from build123d import *

# Parameters (mm, degrees)
BOSS_EXTRUDE1_DEPTH = 3.6
BOSS_EXTRUDE2_DEPTH = 1.5
CUT_EXTRUDE1_DEPTH  = 3.6
BOSS_EXTRUDE5_DEPTH = 3.6
CHAMFER1_SIZE       = 3.6
CHAMFER1_SIZE_2     = 0.062838234
FILLET3_R           = 1
CHAMFER2_SIZE       = 0.6
FILLET4_R           = 0.8


with BuildPart() as part:
    # Sketch1 → Boss-Extrude1 (new body)
    with BuildSketch(Plane(origin=(0, 0, 0), x_dir=(1, 0, 0), z_dir=(0, 1, 0))):
        with BuildLine():
            Line((6, 0), (26.9, 0))
            ThreePointArc((26.9, 0), (31.142640687, 1.757359313), (32.9, 6))
            Line((32.9, 6), (32.9, 17.9))
            ThreePointArc((32.9, 17.9), (31.142640687, 22.142640687), (26.9, 23.9))
            Line((26.9, 23.9), (6, 23.9))
            ThreePointArc((6, 23.9), (1.757359313, 22.142640687), (0, 17.9))
            Line((0, 17.9), (0, 6))
            ThreePointArc((0, 6), (1.757359313, 1.757359313), (6, 0))
        make_face()
    extrude(amount=BOSS_EXTRUDE1_DEPTH)

    # Sketch2 → Boss-Extrude2 (add)
    with BuildSketch(Plane(origin=(0, 3.6, 0), x_dir=(1, 0, 0), z_dir=(0, 1, 0))):
        with BuildLine():
            Line((4.75, 25.15), (28.15, 25.15))
            ThreePointArc((28.15, 25.15), (32.392640687, 23.392640687), (34.15, 19.15))
            Line((34.15, 19.15), (34.15, 4.75))
            ThreePointArc((34.15, 4.75), (32.392640687, 0.507359313), (28.15, -1.25))
            Line((28.15, -1.25), (4.75, -1.25))
            ThreePointArc((4.75, -1.25), (0.507359313, 0.507359313), (-1.25, 4.75))
            Line((-1.25, 4.75), (-1.25, 19.15))
            ThreePointArc((-1.25, 19.15), (0.507359313, 23.392640687), (4.75, 25.15))
        make_face()
    extrude(amount=BOSS_EXTRUDE2_DEPTH)

    # Sketch3 → Cut-Extrude1 (cut)
    with BuildSketch(Plane.XZ):
        with BuildLine():
            Line((25.7, -22.7), (7.2, -22.7))
            ThreePointArc((7.2, -22.7), (2.957359313, -20.942640687), (1.2, -16.7))
            Line((1.2, -16.7), (1.2, -7.2))
            ThreePointArc((1.2, -7.2), (2.957359313, -2.957359313), (7.2, -1.2))
            Line((7.2, -1.2), (25.7, -1.2))
            ThreePointArc((25.7, -1.2), (29.942640687, -2.957359313), (31.7, -7.2))
            Line((31.7, -7.2), (31.7, -16.7))
            ThreePointArc((31.7, -16.7), (29.942640687, -20.942640687), (25.7, -22.7))
        make_face()
    extrude(amount=-CUT_EXTRUDE1_DEPTH, mode=Mode.SUBTRACT)

    # Sketch5 → Boss-Extrude5 (add)
    with BuildSketch(Plane.XZ.offset(-3.6)):
        with BuildLine():
            Line((7.2, -1.2), (8.4, -1.2))
            Line((8.4, -1.2), (8.4, -6.2))
            ThreePointArc((8.4, -6.2), (8.692893219, -6.907106781), (9.4, -7.2))
            Line((9.4, -7.2), (23.5, -7.2))
            ThreePointArc((23.5, -7.2), (24.207106781, -6.907106781), (24.5, -6.2))
            Line((24.5, -6.2), (24.5, -1.2))
            Line((24.5, -1.2), (25.7, -1.2))
            Line((25.7, -1.2), (25.7, -6.2))
            ThreePointArc((25.7, -6.2), (25.992893219, -6.907106781), (26.7, -7.2))
            Line((26.7, -7.2), (31.7, -7.2))
            Line((31.7, -7.2), (31.7, -8.4))
            Line((31.7, -8.4), (26.7, -8.4))
            ThreePointArc((26.7, -8.4), (25.992893219, -8.692893219), (25.7, -9.4))
            Line((25.7, -9.4), (25.7, -14.5))
            ThreePointArc((25.7, -14.5), (25.992893219, -15.207106781), (26.7, -15.5))
            Line((26.7, -15.5), (31.7, -15.5))
            Line((31.7, -15.5), (31.7, -16.7))
            Line((31.7, -16.7), (26.7, -16.7))
            ThreePointArc((26.7, -16.7), (25.992893219, -16.992893219), (25.7, -17.7))
            Line((25.7, -17.7), (25.7, -22.7))
            Line((25.7, -22.7), (24.5, -22.7))
            Line((24.5, -22.7), (24.5, -17.7))
            ThreePointArc((24.5, -17.7), (24.207106781, -16.992893219), (23.5, -16.7))
            Line((23.5, -16.7), (9.4, -16.7))
            ThreePointArc((9.4, -16.7), (8.692893219, -16.992893219), (8.4, -17.7))
            Line((8.4, -17.7), (8.4, -22.7))
            Line((8.4, -22.7), (7.2, -22.7))
            Line((7.2, -22.7), (7.2, -17.7))
            ThreePointArc((7.2, -17.7), (6.907106781, -16.992893219), (6.2, -16.7))
            Line((6.2, -16.7), (1.2, -16.7))
            Line((1.2, -16.7), (1.2, -15.5))
            Line((1.2, -15.5), (6.2, -15.5))
            ThreePointArc((6.2, -15.5), (6.907106781, -15.207106781), (7.2, -14.5))
            Line((7.2, -14.5), (7.2, -9.4))
            ThreePointArc((7.2, -9.4), (6.907106781, -8.692893219), (6.2, -8.4))
            Line((6.2, -8.4), (1.2, -8.4))
            Line((1.2, -8.4), (1.2, -7.2))
            Line((1.2, -7.2), (6.2, -7.2))
            ThreePointArc((6.2, -7.2), (6.907106781, -6.907106781), (7.2, -6.2))
            Line((7.2, -6.2), (7.2, -1.2))
        make_face()
        with BuildLine():
            Line((9.4, -8.4), (23.5, -8.4))
            ThreePointArc((23.5, -8.4), (24.207106781, -8.692893219), (24.5, -9.4))
            Line((24.5, -9.4), (24.5, -14.5))
            ThreePointArc((24.5, -14.5), (24.207106781, -15.207106781), (23.5, -15.5))
            Line((23.5, -15.5), (9.4, -15.5))
            ThreePointArc((9.4, -15.5), (8.692893219, -15.207106781), (8.4, -14.5))
            Line((8.4, -14.5), (8.4, -9.4))
            ThreePointArc((8.4, -9.4), (8.692893219, -8.692893219), (9.4, -8.4))
        make_face(mode=Mode.SUBTRACT)
    extrude(amount=BOSS_EXTRUDE5_DEPTH)

    # Chamfer1
    # the kernel refuses this chamfer: 3.6, 0.062838234 mm, written as the material it takes off along each edge
    with BuildSketch(Plane(origin=(0, 0, -17.9), x_dir=(-0.0006712501823120534, 0.9999997747115711, 0), z_dir=(0, 0, 1))) as chamfer1_piece_1_section:
        Polygon((CHAMFER1_SIZE * 0.999999774712, -CHAMFER1_SIZE * 0.000671250182312), (-CHAMFER1_SIZE_2 * 0.000671250179552, -CHAMFER1_SIZE_2 * 0.999999770599), (0, 0), align=None)
    chamfer1_piece_1 = extrude(amount=11.9, mode=Mode.PRIVATE)
    chamfer1_piece_1 = split(chamfer1_piece_1, bisect_by=Plane(origin=(-0.01902042, 3.6, -11.95), z_dir=(0, -1, 0)), keep=Keep.TOP, mode=Mode.PRIVATE)
    add(chamfer1_piece_1, mode=Mode.SUBTRACT)
    with BuildSketch(Plane(origin=(6, 0, -6), x_dir=(-1, 0, 0), z_dir=(0, 0, -1))) as chamfer1_piece_2_section:
        Polygon((6, CHAMFER1_SIZE), (6 - CHAMFER1_SIZE_2 * 0.999999995888, 0), (6, 0), align=None)
    chamfer1_piece_2 = revolve(axis=Axis((6, 0, -6), (0, 1, 0)), revolution_arc=90, mode=Mode.PRIVATE)
    chamfer1_piece_2 = split(chamfer1_piece_2, bisect_by=Plane(origin=(1.769655981, 3.6, -1.769655981), z_dir=(0, -1, 0)), keep=Keep.TOP, mode=Mode.PRIVATE)
    add(chamfer1_piece_2, mode=Mode.SUBTRACT)
    with BuildSketch(Plane(origin=(6, 0, -17.9), x_dir=(0, 0, -1), z_dir=(1, 0, 0))) as chamfer1_piece_3_section:
        Polygon((6, CHAMFER1_SIZE), (6 - CHAMFER1_SIZE_2 * 0.999999995888, 0), (6, 0), align=None)
    chamfer1_piece_3 = revolve(axis=Axis((6, 0, -17.9), (0, 1, 0)), revolution_arc=90, mode=Mode.PRIVATE)
    chamfer1_piece_3 = split(chamfer1_piece_3, bisect_by=Plane(origin=(1.769655981, 3.6, -22.130344019), z_dir=(0, -1, 0)), keep=Keep.TOP, mode=Mode.PRIVATE)
    add(chamfer1_piece_3, mode=Mode.SUBTRACT)
    with BuildSketch(Plane(origin=(6, 0, 0), x_dir=(0, 0.9999997747115711, 0.0006712501823120534), z_dir=(1, 0, 0))) as chamfer1_piece_4_section:
        Polygon((CHAMFER1_SIZE * 0.999999774712, -CHAMFER1_SIZE * 0.000671250182312), (-CHAMFER1_SIZE_2 * 0.000671250179552, -CHAMFER1_SIZE_2 * 0.999999770599), (0, 0), align=None)
    chamfer1_piece_4 = extrude(amount=20.9, mode=Mode.PRIVATE)
    chamfer1_piece_4 = split(chamfer1_piece_4, bisect_by=Plane(origin=(16.45, 3.6, 0.01902042), z_dir=(0, -1, 0)), keep=Keep.TOP, mode=Mode.PRIVATE)
    add(chamfer1_piece_4, mode=Mode.SUBTRACT)
    with BuildSketch(Plane(origin=(26.9, 0, -23.9), x_dir=(0, 0.9999997747115711, -0.0006712501823119971), z_dir=(-1, 0, 0))) as chamfer1_piece_5_section:
        Polygon((CHAMFER1_SIZE * 0.999999774712, -CHAMFER1_SIZE * 0.000671250182312), (-CHAMFER1_SIZE_2 * 0.000671250179552, -CHAMFER1_SIZE_2 * 0.999999770599), (0, 0), align=None)
    chamfer1_piece_5 = extrude(amount=20.9, mode=Mode.PRIVATE)
    chamfer1_piece_5 = split(chamfer1_piece_5, bisect_by=Plane(origin=(16.45, 3.6, -23.91902042), z_dir=(0, -1, 0)), keep=Keep.TOP, mode=Mode.PRIVATE)
    add(chamfer1_piece_5, mode=Mode.SUBTRACT)
    with BuildSketch(Plane(origin=(26.9, 0, -6), x_dir=(0, 0, 1), z_dir=(-1, 0, 0))) as chamfer1_piece_6_section:
        Polygon((6, CHAMFER1_SIZE), (6 - CHAMFER1_SIZE_2 * 0.999999995888, 0), (6, 0), align=None)
    chamfer1_piece_6 = revolve(axis=Axis((26.9, 0, -6), (0, 1, 0)), revolution_arc=90, mode=Mode.PRIVATE)
    chamfer1_piece_6 = split(chamfer1_piece_6, bisect_by=Plane(origin=(31.130344019, 3.6, -1.769655981), z_dir=(0, -1, 0)), keep=Keep.TOP, mode=Mode.PRIVATE)
    add(chamfer1_piece_6, mode=Mode.SUBTRACT)
    with BuildSketch(Plane(origin=(26.9, 0, -17.9), x_dir=(1, 0, 0), z_dir=(0, 0, 1))) as chamfer1_piece_7_section:
        Polygon((6, CHAMFER1_SIZE), (6 - CHAMFER1_SIZE_2 * 0.999999995888, 0), (6, 0), align=None)
    chamfer1_piece_7 = revolve(axis=Axis((26.9, 0, -17.9), (0, 1, 0)), revolution_arc=90, mode=Mode.PRIVATE)
    chamfer1_piece_7 = split(chamfer1_piece_7, bisect_by=Plane(origin=(31.130344019, 3.6, -22.130344019), z_dir=(0, -1, 0)), keep=Keep.TOP, mode=Mode.PRIVATE)
    add(chamfer1_piece_7, mode=Mode.SUBTRACT)
    with BuildSketch(Plane(origin=(32.9, 0, -6), x_dir=(0.000671250182312946, 0.9999997747115711, 0), z_dir=(0, 0, -1))) as chamfer1_piece_8_section:
        Polygon((CHAMFER1_SIZE * 0.999999774712, -CHAMFER1_SIZE * 0.000671250182313), (-CHAMFER1_SIZE_2 * 0.000671250179553, -CHAMFER1_SIZE_2 * 0.999999770599), (0, 0), align=None)
    chamfer1_piece_8 = extrude(amount=11.9, mode=Mode.PRIVATE)
    chamfer1_piece_8 = split(chamfer1_piece_8, bisect_by=Plane(origin=(32.91902042, 3.6, -11.95), z_dir=(0, -1, 0)), keep=Keep.TOP, mode=Mode.PRIVATE)
    add(chamfer1_piece_8, mode=Mode.SUBTRACT)

    # Fillet3
    fillet3_edges = [part.edges().sort_by_distance(p)[0] for p in [
        (1.2, 1.8, -8.4),
        (1.2, 1.8, -15.5),
        (8.4, 1.8, -22.7),
        (24.5, 1.8, -22.7),
        (31.7, 1.8, -15.5),
        (31.7, 1.8, -8.4),
        (24.5, 1.8, -1.2),
        (8.4, 1.8, -1.2),
        (7.2, 1.8, -22.7),
        (1.2, 1.8, -16.7),
        (1.2, 1.8, -7.2),
        (7.2, 1.8, -1.2),
        (25.7, 1.8, -1.2),
        (31.7, 1.8, -7.2),
        (31.7, 1.8, -16.7),
        (25.7, 1.8, -22.7),
    ]]
    fillet(fillet3_edges, radius=FILLET3_R)

    # Chamfer2
    chamfer2_edges = [part.edges().sort_by_distance(p)[0] for p in [
        (0.507359313, 5.1, -0.507359313),
        (16.45, 5.1, 1.25),
        (32.392640687, 5.1, -0.507359313),
        (34.15, 5.1, -11.95),
        (32.392640687, 5.1, -23.392640687),
        (16.45, 5.1, -25.15),
        (0.507359313, 5.1, -23.392640687),
        (-1.25, 5.1, -11.95),
    ]]
    chamfer(chamfer2_edges, length=CHAMFER2_SIZE)

    # Fillet4
    fillet4_edges = [part.edges().sort_by_distance(p)[0] for p in [
        (16.45, 4.5, -25.15),
        (0.507359313, 4.5, -23.392640687),
        (32.392640687, 4.5, -23.392640687),
        (-1.25, 4.5, -11.95),
        (34.15, 4.5, -11.95),
        (0.507359313, 4.5, -0.507359313),
        (32.392640687, 4.5, -0.507359313),
        (16.45, 4.5, 1.25),
    ]]
    fillet(fillet4_edges, radius=FILLET4_R)


solid = part.part
Source: CAD feature listing. Evaluate the final solid. Frame: model axes, mm. A direction names the side the tool comes from. Give positions to 0.01 mm unless a question says otherwise; leave off trailing zeros. Write each loop counter-clockwise with the first axis right and the second up, starting at its lowest first coordinate (ties: lowest second). Pieces come first, ordered by that corner, then holes. Notation, with made-up numbers: (-6, 51) -> (2, 51) arc R18 ccw to (2, 79) -> close; hole circle Ø5 at (70, -29.5). An arc over 180 degrees is marked (long way). Write item = value, one per line.
Q1. Reachability of faces 1 (the face through (0.876, 4.96, -0.79)), 2 (the face through (1.83, 1.77, -22.17)), 3 (the face through (8.685, 1.825, -6.899)) from +Z, -Z, +X, -X, +Y, -Y: full face, straight path, thin tool, end or side. Return the list, or none.
Here are the results:
face_1 = +Z, -X, +Y
face_2 = -Z, -X, -Y
face_3 = -Y
Q2. Cut plane A-A on x = 25. Return loops of the section in (y, z), then the cut area to 3 significant figures.
Here are the results:
outline = (0, -23.84) -> (3.6, -23.9) -> (3.6, -25.15) -> (4.17, -25.15) arc R0.8 ccw to (4.73, -24.92) -> (5.1, -24.55) -> (5.1, 0.65) -> (4.73, 1.02) arc R0.8 ccw to (4.17, 1.25) -> (3.6, 1.25) -> (3.6, 0) -> (0, -0.06) -> close
area = 125 mm²
Q3. Cut plane B-B on z = -10. Return loops of the section in (x, y).
Here are the results:
outline = (-1.25, 3.6) -> (0, 3.6) -> (0.06, 0) -> (1.2, 0) -> (1.2, 3.6) -> (7.2, 3.6) -> (7.2, 0) -> (8.4, 0) -> (8.4, 3.6) -> (24.5, 3.6) -> (24.5, 0) -> (25.7, 0) -> (25.7, 3.6) -> (31.7, 3.6) -> (31.7, 0) -> (32.84, 0) -> (32.9, 3.6) -> (34.15, 3.6) -> (34.15, 4.17) arc R0.8 ccw to (33.92, 4.73) -> (33.55, 5.1) -> (-0.65, 5.1) -> (-1.02, 4.73) arc R0.8 ccw to (-1.25, 4.17) -> close
Q4. Mould query, pull axis Z, two halves, no side actions, for faces 4 (the face through (5, 3.6, -19)), 5 (the face through (0.554, 3.88, -0.461)), 6 (the face through (32.346, 3.88, -23.439)). Classes: +Z half, -Z half, draft (parallel to the pull), parting line (faces both ways), or undercut.
Here are the results:
face_4 = undercut
face_5 = +Z half
face_6 = -Z half
Q5. First-contact query: pin 1 (8 mm diameter, centred on x = 21.5, z = -16.5, fed in from -Y); pin 2 (3.5 mm diameter, centred on x = 17, z = -12.5, fed in from -Y); pin 3 (1.5 mm diameter, centred on x = 14, y = 1, fed in from +Z); pin 4 (3 mm diameter, centred on y = 1.5, z = -11, fed in from -X). Flat tips, straight axial feed; report the tip coordinate or a pass-through.
Here are the results:
pin_1 = 0
pin_2 = 3.6
pin_3 = -0.03
pin_4 = 0.01
Q6. Cut plane D-D on x = 18. Return loops of the section in (y, z).
Here are the results:
outline = (0, -23.84) -> (3.6, -23.9) -> (3.6, -25.15) -> (4.17, -25.15) arc R0.8 ccw to (4.73, -24.92) -> (5.1, -24.55) -> (5.1, 0.65) -> (4.73, 1.02) arc R0.8 ccw to (4.17, 1.25) -> (3.6, 1.25) -> (3.6, 0) -> (0, -0.06) -> (0, -1.2) -> (3.6, -1.2) -> (3.6, -7.2) -> (0, -7.2) -> (0, -8.4) -> (3.6, -8.4) -> (3.6, -15.5) -> (0, -15.5) -> (0, -16.7) -> (3.6, -16.7) -> (3.6, -22.7) -> (0, -22.7) -> close
Q7. Cut plane C-C on y = 2.65. State how many separate pieces and enclosed holes the cut face has, then the cut area to 3 significant figures.
Here are the results:
separate_pieces = 1
enclosed_holes = 9
area = 255 mm²
Q8. Line query: line 1 (Z direction, x = 11, y = 3.1); line 2 (X direction, y = 2.95, z = -10.5); line 3 (X direction, y = 1.8, z = -20.75). Output: solid intervals per line, ascending. Write a range as from..to.
Here are the results:
line_1 = -23.89..-22.7, -16.7..-15.5, -8.4..-7.2, -1.2..-0.01
line_2 = 0.01..1.2, 7.2..8.4, 24.5..25.7, 31.7..32.89
line_3 = 0.76..2.77, 7.2..8.4, 24.5..25.7, 30.13..32.14
